Source: CAD feature listing. Evaluate the final solid. Frame: model axes, mm. A direction names the side the tool comes from. Round coordinates to 2 decimals unless told otherwise and drop trailing zeros. Loops run counter-clockwise (first coordinate to the right, second up) from the corner with the lowest first, then second, coordinate; pieces in that order, holes last. Notation, with made-up numbers: M 12.5,45 L 52.5,45 A12 cw 52.5,58 Z; hole C 84.25,-25.5 d3. An arc over 180 degrees is marked long. One line per item, written item: value.
from build123d import *

# Parameters (mm, degrees)
SKETCH_1_R             = 8
EXTRUDE_1_DEPTH        = 161.6
HOLE_WIZARD_M103_D     = 8.5
HOLE_WIZARD_M103_DEPTH = 35
HOLE_WIZARD_M103_TIP   = 2.553657631
HOLE_WIZARD_M104_D     = 8.5
HOLE_WIZARD_M104_DEPTH = 35
HOLE_WIZARD_M104_TIP   = 2.553657631


with BuildPart() as part:
    # Эскиз1 → Бобышка-Вытянуть1 (new body)
    with BuildSketch(Plane.XY):
        with Locations((100, -317)):
            Circle(SKETCH_1_R)
    extrude(amount=EXTRUDE_1_DEPTH)

    # Отверстие обработанное метчиком M103
    with Locations(Plane.XY.offset(161.6)):
        with Locations((100, -317)):
            Hole(HOLE_WIZARD_M103_D / 2, depth=HOLE_WIZARD_M103_DEPTH)
            with Locations((0, 0, -(HOLE_WIZARD_M103_DEPTH + HOLE_WIZARD_M103_TIP / 2))):  # 118° drill point
                Cone(0, HOLE_WIZARD_M103_D / 2, HOLE_WIZARD_M103_TIP, mode=Mode.SUBTRACT)

    # Отверстие обработанное метчиком M104
    with Locations(Plane(origin=(0, 0, 0), x_dir=(-1, 0, 0), z_dir=(0, 0, -1))):
        with Locations((-100, -317)):
            Hole(HOLE_WIZARD_M104_D / 2, depth=HOLE_WIZARD_M104_DEPTH)
            with Locations((0, 0, -(HOLE_WIZARD_M104_DEPTH + HOLE_WIZARD_M104_TIP / 2))):  # 118° drill point
                Cone(0, HOLE_WIZARD_M104_D / 2, HOLE_WIZARD_M104_TIP, mode=Mode.SUBTRACT)


solid = part.part
1. Reachability of faces 4 (the face through (99.447, -312.786, 17.745)), 5 (the face through (103.4, -320.4, 161.6)), 6 (the face through (100.553, -312.786, 143.855)) from +Z, -Z, +X, -X, +Y, -Y: full face, straight path, thin tool, end or side. Return the list, or none.
Report:
face 4: -Z
face 5: +Z, +X, -X, +Y, -Y
face 6: +Z
2. Section query B-B (z = 87). Return the cut outline in (x, y).
Report:
outline: C 100,-317 d16
3. Ray query, line 1 (Y direction, x = 100, z = 145.5); line 2 (Y direction, x = 98, z = 154); line 3 (X direction, y = -316, z = 135.5). Return the intervals inside material, ascending. Write a range as [from, to].
Report:
line 1: y = [-325, -321.25], [-312.75, -309]
line 2: y = [-324.75, -320.75], [-313.25, -309.25]
line 3: x = [92.06, 95.87], [104.13, 107.94]
4. Section query A-A (z = 15.5). Return the cut outline in (x, y), and give its area (3 significant figures).
Report:
outline: C 100,-317 d16; hole C 100,-317 d8.5
area: 144 mm2
5. Section query C-C (y = -323.25). Return the cut outline in (x, z), and give its area (3 significant figures).
Report:
outline: M 95.01,0 L 104.99,0 L 104.99,161.6 L 95.01,161.6 Z
area: 1,610 mm2
6. Pin query (flat end, axial travel): pin 1 (1 mm diameter, centred on x = 96, z = 99, fed in from -Y); pin 2 (8 mm diameter, centred on y = -323.5, z = 80, fed in from +X); pin 3 (4 mm diameter, centred on y = -320, z = 123, fed in from -X). Return the tip coordinate at first contact, or that it passes through.
Report:
pin 1: stops at y = -324.19
pin 2: stops at x = 107.6
pin 3: stops at x = 92.06
7. Pull-direction query (X, two-part tool) for faces 1 (the face through (103.4, -320.4, 0)), 2 (the face through (99.26, -316.97, 124.49)), 3 (the face through (98.959, -309.068, 79.669)); classes: released by +X, released by -X, zero draft, split by the parting line, or undercut.
Report:
face 1: zero draft
face 2: undercut
face 3: split by the parting line
